Source: CAD feature listing. Evaluate the final solid. Frame: model axes, mm. Face numbers are marked on the shaded views. A direction names the side the tool comes from. Round coordinates to 2 decimals unless told otherwise and drop trailing zeros. Order: outer loops, then holes, each group sorted by start corner. A loop starts at its lowest first (then second) coordinate and runs counter-clockwise, first axis right, second up. Notation, with made-up numbers: (65, -20.5) - (121, -20.5) arc R22 ccw to (121, 5.5) - close; hole circle Ø4 at (65.5, -27.75). An arc over 180 degrees is marked (long way). Use one line per item in the form item = value. Start each with the question number.
Q1. Set-up query: the marked faces 4 and 5. Return all of +Z, -Z, +X, -X, +Y, -Y with unobstructed straight access to the full face (end or side cutting, diameter ignored); none if empty.
Q2. Cut plane C-C, the plane x = 2.5. Return the cut outline in (y, z).
Q3. Draft query along X for the marked faces 1, 2 and 3. Return one class per face: released by +X, released by -X, zero draft, split by the parting line, or undercut.
Q4. Cut plane B-B, the plane y = 7.5. Return the cut outline in (x, z), and give its area (3 significant figures).
Q5. Cut plane A-A, the plane z = 7.5. Return the cut outline in (x, y).
Q6. Cut plane D-D, the plane z = 14.5. Return the cut outline in (x, y), and give its area (3 significant figures).
Q7. Ray query, line 1 (Y direction, x = 1.75, z = 6.5); line 2 (X direction, y = 7.5, z = 10.25); line 3 (Z direction, x = 2, y = 0.75). Return the intervals inside material, ascending. Write a range as [from, to].
Autodesk Fusion 360 part; units mm, degrees
sketch "Sketch2" plane through (0, 0, 0) normal (0, 0, 1) x (1, 0, 0)
  line L0 (0, 0) -> (4.6, 0)
  line L1 (4.6, 0) -> (4.6, 12.1)
  line L2 (4.6, 12.1) -> (0, 12.1)
  line L3 (0, 12.1) -> (0, 0)
  line L4 (-1.5, 13.6) -> (6.1, 13.6)
  line L5 (6.1, 13.6) -> (6.1, -1.5)
  line L6 (6.1, -1.5) -> (-1.5, -1.5)
  line L7 (-1.5, -1.5) -> (-1.5, 13.6)
  dimension "d1" = 4.6
  dimension "d2" = 12.1
  dimension "d3" = 1.5
  dimension "d4" = 1.5
  dimension "d5" = 1.5
  dimension "d6" = 1.5
extrude "Extrude1" add sketch "Sketch2" along normal blind 14
sketch "Sketch3" plane through (0, 0, 14) normal (0, 0, 1) x (-1, 0, 0)
  line L0 (0, 0) -> (0, -12.1)
  line L1 (0, -12.1) -> (-4.6, -12.1)
  line L2 (-4.6, -12.1) -> (-4.6, 0)
  line L3 (-4.6, 0) -> (0, 0)
  line L4 (1.5, 1.5) -> (-6.1, 1.5)
  line L5 (-6.1, 1.5) -> (-6.1, -13.6)
  line L6 (-6.1, -13.6) -> (1.5, -13.6)
  line L7 (1.5, -13.6) -> (1.5, 1.5)
  line L8 (1.5, -13.6) -> (-6.1, -13.6)
  line L9 (-6.1, -13.6) -> (-6.1, 1.5)
  line L10 (-6.1, 1.5) -> (1.5, 1.5)
  line L11 (1.5, 1.5) -> (1.5, -13.6)
extrude "Extrude2" add sketch "Sketch3" along normal blind 3 contours L0 L1 L2 L3 | L4 L5 L6 L7 L8 L9 L10 L11
fillet "Fillet1" radius 3 4 edges at (-1.5, 13.6, 8.5) (-1.5, -1.5, 8.5) (6.1, -1.5, 8.5) (6.1, 13.6, 8.5)
fillet "Fillet1" radius 2 4 edges at (6.1, 6.05, 17) (2.3, -1.5, 17) (-1.5, 6.05, 17) (2.3, 13.6, 17)
equation "d4 = d3"
equation "d5 = d4"
equation "d6 = d3"
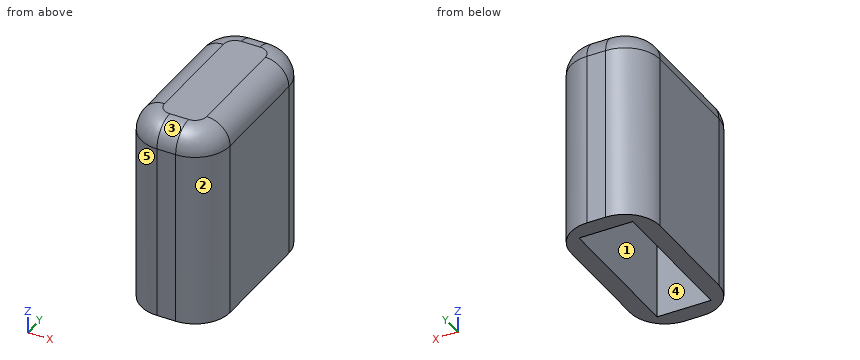
Completed:
q1.face_4 = -Z
q1.face_5 = +Z, -Z, -X, -Y
q2.outline = (-1.5, 0) - (0, 0) - (0, 14) - (12.1, 14) - (12.1, 0) - (13.6, 0) - (13.6, 15) arc R2 ccw to (11.6, 17) - (0.5, 17) arc R2 ccw to (-1.5, 15) - close
q3.face_1 = undercut
q3.face_2 = released by +X
q3.face_3 = zero draft
q4.outline = (-1.5, 0) - (0, 0) - (0, 14) - (4.6, 14) - (4.6, 0) - (6.1, 0) - (6.1, 15) arc R2 ccw to (4.1, 17) - (0.5, 17) arc R2 ccw to (-1.5, 15) - close
q4.area = 63.1 mm2
q5.outline = (-1.5, 1.5) arc R3 ccw to (1.5, -1.5) - (3.1, -1.5) arc R3 ccw to (6.1, 1.5) - (6.1, 10.6) arc R3 ccw to (3.1, 13.6) - (1.5, 13.6) arc R3 ccw to (-1.5, 10.6) - close; hole (0, 0) - (4.6, 0) - (4.6, 12.1) - (0, 12.1) - close
q6.outline = (-1.5, 1.5) arc R3 ccw to (1.5, -1.5) - (3.1, -1.5) arc R3 ccw to (6.1, 1.5) - (6.1, 10.6) arc R3 ccw to (3.1, 13.6) - (1.5, 13.6) arc R3 ccw to (-1.5, 10.6) - close
q6.area = 107 mm2
q7.line_1 = [-1.5, 0], [12.1, 13.6]
q7.line_2 = [-1.5, 0], [4.6, 6.1]
q7.line_3 = [14, 17]
